Solid Edge part; units mm, degrees
sketch "Sketch1" plane through (0, 0, 0) normal (0, -1, 0) x (1, 0, 0)
  line L0 (4, 0) -> (1.8, 0)
  line L1 (1.8, 0) -> (1.8, -1.4)
  line L2 (1.8, -1.4) -> (2, -1.4)
  line L3 (2, -1.4) -> (2, -20)
  line L4 (2, -20) -> (0, -20)
  arc A0 (0, 3.1) -> (4, 2.0282) centre (0, -4.9) cw
  line L5 (4, 0) -> (4, 2.0282)
  dimension "D1" = 1.8
  dimension "D2" = 1.8
revolve "RevolvedProtrusion1" add sketch "Sketch1" angle 360 about axis through (0, 0, -6) along (0, 0, 1)
cosmetic_thread "Thread1"
chamfer "Chamfer_1" distance 0.4 angle 45 1 edges at (-2, 0, -20)
fillet "Round1" radius 0.2 2 edges at (-1.8, 0, -1.4) (-1.8, 0, 0)
fillet "Round_3" radius 1 1 edges at (-4, 0, 2.0282)
sketch "Sketch2" plane through (0, 0, 3.1) normal (0, 0, 1) x (1, 0, 0)
  line L0 (-0.5, 0.5) -> (-0.5, 2.3)
  line L1 (-0.5, 2.3) -> (0.5, 2.3)
  line L2 (0.5, 2.3) -> (0.5, 0.5)
  line L3 (0.5, 0.5) -> (2.3, 0.5)
  line L4 (2.3, 0.5) -> (2.3, -0.5)
  line L5 (2.3, -0.5) -> (0.5, -0.5)
  line L6 (0.5, -0.5) -> (0.5, -2.3)
  line L7 (0.5, -2.3) -> (-0.5, -2.3)
  line L8 (-0.5, -2.3) -> (-0.5, -0.5)
  line L9 (-0.5, -0.5) -> (-2.3, -0.5)
  line L10 (-2.3, -0.5) -> (-2.3, 0.5)
  line L11 (-2.3, 0.5) -> (-0.5, 0.5)
  dimension "D1" = 0.5
extrude "ExtrudedCutout_2" cut sketch "Sketch2" against normal blind 2.3
properties material "Galvanized steel"
Part model, mm, in its own coordinate system. A direction names the side the tool comes from. Round coordinates to 2 decimals unless told otherwise and drop trailing zeros. Write each loop counter-clockwise with the first axis right and the second up, starting at its lowest first coordinate (ties: lowest second). Pieces come first, ordered by that corner, then holes. Notation, with made-up numbers: (13.5, 79.25) -> (61.5, 79.25) arc R25 ccw to (61.5, 95.25) -> close; hole circle Ø8 at (9, 31.5). An arc over 180 degrees is marked (long way). Return JSON: item names as keys, results as strings. Group by question number.
Q1. Pin check, flat tips, straight feed: pin 1 (0.5 mm diameter, centred on x = 0, z = 2, fed in from -Y); pin 2 (1.4 mm diameter, centred on x = -1, y = 0, fed in from +Z); pin 3 (4 mm diameter, centred on y = -1, z = -7, fed in from +X). Stop position of each tip, or through.
Q2. Saw through at A-A on z = -12. Write the cut outline in (x, y).
Q3. Mould opens along Y. For faces 1 (the cylindrical face through (0, 2, -11)), 2 (the flat face through (0, 0, -20)), 3 (the flat face through (-1, 0.5, 2)), 4 (the flat face through (1, 0.5, 2)) say: pulls with the +Y half, pulls with the -Y half, needs draft (parallel to the pull), parting line crosses it, or undercut.
Q4. Probe L1, parallel to X at y = -1.5, z = 1.5; L2, parallel to Z at x = 0, y = 3; L3, parallel to Z at x = 0.75, y = -2.5. List the from-to ranges inside material, lowest first. Write a range as [from, to].
Q5. Which spindle directions (+Z, -Z, +X, -X, +Y, -Y) get a long thin tool onto all of the face, cutting with end or side? Do faces 5 (the flat face through (0.5, -1, 2)), 6 (the cylindrical face through (-0.867, -3.905, 0.722)), 7 (the cylindrical face through (1.717, -0.541, -0.707)). Say none if no direction does.
Answer:
{
 "1": {"pin 1": "y = -3.95", "pin 2": "z = 3.07", "pin 3": "x = 2"},
 "2": {"outline": "circle Ø4 at (0, 0)"},
 "3": {"face 1": "parting line crosses it", "face 2": "needs draft", "face 3": "undercut", "face 4": "undercut"},
 "4": {"L1": "[-3.71, -0.5], [0.5, 3.71]", "L2": "[0, 2.52]", "L3": "[0, 2.66]"},
 "5": {"face 5": "+Z", "face 6": "+Z, -Z", "face 7": "none"}
}
